from build123d import *

# Parameters (mm, degrees)
BOSS_EXTRUDE1_DEPTH             = 47
SKETCH3_W                       = 84.887301628
SKETCH3_H                       = 42
CUT_EXTRUDE1_DEPTH              = 40
SKETCH4_W                       = 55.556349186
SKETCH4_H                       = 42
CUT_EXTRUDE2_DEPTH              = 10.556349186
SKETCH5_W                       = 55.556349186
SKETCH5_H                       = 42
CUT_EXTRUDE3_DEPTH              = 10.556349186
CUT_EXTRUDE5_REACH              = 130.666
SKETCH7_W                       = 10
SKETCH7_H                       = 18
CUT_EXTRUDE6_REACH              = 135.004
SKETCH8_R                       = 6.5
BOSS_EXTRUDE2_DEPTH             = 5
CUT_EXTRUDE7_REACH              = 105.666
CUT_EXTRUDE7_START              = -5
SKETCH11_W                      = 106
SKETCH11_H                      = 47
BOSS_EXTRUDE3_DEPTH             = 5
CUT_EXTRUDE8_REACH              = 91.961
CUT_EXTRUDE9_REACH              = 91.961
SKETCH14_W                      = 75
SKETCH14_H                      = 27
CUT_EXTRUDE10_REACH             = 136.852
SKETCH16_R                      = 2.1
CUT_EXTRUDE10_DIRECTION_2_DEPTH = 135.851770474
CUT_EXTRUDE11_REACH             = 136.852
SKETCH17_R                      = 2.1


with BuildPart() as part:
    # Sketch1 → Boss-Extrude1 (new body)
    with BuildSketch(Plane(origin=(0, 0, 0), x_dir=(1, 0, 0), z_dir=(0, 1, 0))):
        Polygon((-42.443650814, 0), (42.443650814, 0), (58, 15.556349186), (58, -45), (-58, -45), (-58, 15.556349186), align=None)
    extrude(amount=BOSS_EXTRUDE1_DEPTH)

    # Sketch3 → Cut-Extrude1 (cut)
    with BuildSketch(Plane(origin=(0, 0, 0), x_dir=(-1, 0, 0), z_dir=(0, 0, -1))):
        with Locations((0, 21)):
            Rectangle(SKETCH3_W, SKETCH3_H)
    extrude(amount=-CUT_EXTRUDE1_DEPTH, mode=Mode.SUBTRACT)

    # Sketch4 → Cut-Extrude2 (cut)
    with BuildSketch(Plane.ZY.offset(-42.443650814)):
        with Locations((12.221825407, 21)):
            Rectangle(SKETCH4_W, SKETCH4_H)
    extrude(amount=-CUT_EXTRUDE2_DEPTH, mode=Mode.SUBTRACT)

    # Sketch5 → Cut-Extrude3 (cut)
    with BuildSketch(Plane(origin=(-42.443650814, 0, 0), x_dir=(0, 0, -1), z_dir=(1, 0, 0))):
        with Locations((-12.221825407, 21)):
            Rectangle(SKETCH5_W, SKETCH5_H)
    extrude(amount=-CUT_EXTRUDE3_DEPTH, mode=Mode.SUBTRACT)

    # Sketch7 → Cut-Extrude5 (cut, up to next)
    with BuildSketch(Plane.ZY.offset(-53), mode=Mode.PRIVATE) as cut_extrude5_sk1:
        with Locations((8, 13)):
            Rectangle(SKETCH7_W, SKETCH7_H)
    cut_extrude5_tool1 = extrude(cut_extrude5_sk1.sketch, amount=-CUT_EXTRUDE5_REACH, mode=Mode.PRIVATE) & part.part
    add(cut_extrude5_tool1.solids().sort_by_distance((53, 13, 8))[0], mode=Mode.SUBTRACT)

    # Sketch8 → Cut-Extrude6 (cut, up to next)
    with BuildSketch(Plane.ZY.offset(58), mode=Mode.PRIVATE) as cut_extrude6_sk1:
        with Locations((8.5, 12.301549083)):
            Circle(SKETCH8_R)
    cut_extrude6_tool1 = extrude(cut_extrude6_sk1.sketch, amount=-CUT_EXTRUDE6_REACH, mode=Mode.PRIVATE) & part.part
    add(cut_extrude6_tool1.solids().sort_by_distance((-58, 12.301549, 8.5))[0], mode=Mode.SUBTRACT)

    # Sketch10 → Boss-Extrude2 (add)
    with BuildSketch(Plane(origin=(0, 47, 0), x_dir=(1, 0, 0), z_dir=(0, 1, 0))):
        Polygon((58, -45), (-58, -45), (-58, 15.556349186), (-42.443650814, 0), (42.443650814, 0), (58, 15.556349186), align=None)
    extrude(amount=BOSS_EXTRUDE2_DEPTH)

    # Sketch11 → Cut-Extrude7 (cut, up to next)
    with BuildSketch(Plane.XY.offset(45).offset(CUT_EXTRUDE7_START), mode=Mode.PRIVATE) as cut_extrude7_sk1:
        with Locations((0, 23.5)):
            Rectangle(SKETCH11_W, SKETCH11_H)
    cut_extrude7_tool1 = extrude(cut_extrude7_sk1.sketch, amount=-CUT_EXTRUDE7_REACH, mode=Mode.PRIVATE) & part.part
    add(cut_extrude7_tool1.solids().sort_by_distance((0, 23.5, 40))[0], mode=Mode.SUBTRACT)

    # Sketch12 → Boss-Extrude3 (add)
    with BuildSketch(Plane(origin=(0, 52, 0), x_dir=(1, 0, 0), z_dir=(0, 1, 0))):
        Polygon((58, 15.556349186), (42.443650814, 0), (-42.443650814, 0), (-58, 15.556349186), align=None)
    extrude(amount=-BOSS_EXTRUDE3_DEPTH)

    # Sketch13 → Cut-Extrude8 (cut, up to next)
    with BuildSketch(Plane(origin=(0, 52, 0), x_dir=(1, 0, 0), z_dir=(0, 1, 0)), mode=Mode.PRIVATE) as cut_extrude8_sk1:
        with BuildLine():
            Line((26, 7.556349186), (26, 15.556349186))
            ThreePointArc((26, 15.556349186), (31, 20.556349186), (36, 15.556349186))
            Line((36, 15.556349186), (36, 7.556349186))
            ThreePointArc((36, 7.556349186), (31, 2.556349186), (26, 7.556349186))
        make_face()
    cut_extrude8_tool1 = extrude(cut_extrude8_sk1.sketch, amount=-CUT_EXTRUDE8_REACH, mode=Mode.PRIVATE) & part.part
    # Sketch13 → Cut-Extrude8 (cut, up to next)
    with BuildSketch(Plane(origin=(0, 52, 0), x_dir=(1, 0, 0), z_dir=(0, 1, 0)), mode=Mode.PRIVATE) as cut_extrude8_sk2:
        with BuildLine():
            Line((11.5, 7.556349186), (11.5, 15.556349186))
            ThreePointArc((11.5, 15.556349186), (15, 19.056349186), (18.5, 15.556349186))
            Line((18.5, 15.556349186), (18.5, 7.556349186))
            ThreePointArc((18.5, 7.556349186), (15, 4.056349186), (11.5, 7.556349186))
        make_face()
    cut_extrude8_tool2 = extrude(cut_extrude8_sk2.sketch, amount=-CUT_EXTRUDE8_REACH, mode=Mode.PRIVATE) & part.part
    # Sketch13 → Cut-Extrude8 (cut, up to next)
    with BuildSketch(Plane(origin=(0, 52, 0), x_dir=(1, 0, 0), z_dir=(0, 1, 0)), mode=Mode.PRIVATE) as cut_extrude8_sk3:
        with BuildLine():
            Line((-15.5, 7.556349186), (-15.5, 15.556349186))
            ThreePointArc((-15.5, 15.556349186), (-12, 19.056349186), (-8.5, 15.556349186))
            Line((-8.5, 15.556349186), (-8.5, 7.556349186))
            ThreePointArc((-8.5, 7.556349186), (-12, 4.056349186), (-15.5, 7.556349186))
        make_face()
    cut_extrude8_tool3 = extrude(cut_extrude8_sk3.sketch, amount=-CUT_EXTRUDE8_REACH, mode=Mode.PRIVATE) & part.part
    # Sketch13 → Cut-Extrude8 (cut, up to next)
    with BuildSketch(Plane(origin=(0, 52, 0), x_dir=(1, 0, 0), z_dir=(0, 1, 0)), mode=Mode.PRIVATE) as cut_extrude8_sk4:
        with BuildLine():
            Line((-34.5, 7.556349186), (-34.5, 15.556349186))
            ThreePointArc((-34.5, 15.556349186), (-31, 19.056349186), (-27.5, 15.556349186))
            Line((-27.5, 15.556349186), (-27.5, 7.556349186))
            ThreePointArc((-27.5, 7.556349186), (-31, 4.056349186), (-34.5, 7.556349186))
        make_face()
    cut_extrude8_tool4 = extrude(cut_extrude8_sk4.sketch, amount=-CUT_EXTRUDE8_REACH, mode=Mode.PRIVATE) & part.part
    add(cut_extrude8_tool1.solids().sort_by_distance((31, 52, -11.556349))[0], mode=Mode.SUBTRACT)
    add(cut_extrude8_tool2.solids().sort_by_distance((15, 52, -11.556349))[0], mode=Mode.SUBTRACT)
    add(cut_extrude8_tool3.solids().sort_by_distance((-12, 52, -11.556349))[0], mode=Mode.SUBTRACT)
    add(cut_extrude8_tool4.solids().sort_by_distance((-31, 52, -11.556349))[0], mode=Mode.SUBTRACT)

    # Sketch14 → Cut-Extrude9 (cut, up to next)
    with BuildSketch(Plane(origin=(0, 52, 0), x_dir=(1, 0, 0), z_dir=(0, 1, 0)), mode=Mode.PRIVATE) as cut_extrude9_sk1:
        with Locations((0, -26.5)):
            Rectangle(SKETCH14_W, SKETCH14_H)
    cut_extrude9_tool1 = extrude(cut_extrude9_sk1.sketch, amount=-CUT_EXTRUDE9_REACH, mode=Mode.PRIVATE) & part.part
    add(cut_extrude9_tool1.solids().sort_by_distance((0, 52, 26.5))[0], mode=Mode.SUBTRACT)

    # Sketch16 → Cut-Extrude10 (cut, up to next)
    with BuildSketch(Plane(origin=(58, 0, 0), x_dir=(0, 0, -1), z_dir=(1, 0, 0)), mode=Mode.PRIVATE) as cut_extrude10_sk1:
        with Locations(Location((8.456349186, 10, 0), (0, 0, 180))):
            Circle(SKETCH16_R)
    cut_extrude10_tool1 = extrude(cut_extrude10_sk1.sketch, amount=-CUT_EXTRUDE10_REACH, mode=Mode.PRIVATE) & part.part
    add(cut_extrude10_tool1.solids().sort_by_distance((58, 10, -8.456349))[0], mode=Mode.SUBTRACT)

    # Sketch16 → Cut-Extrude10 direction 2 (cut)
    with BuildSketch(Plane(origin=(58, 0, 0), x_dir=(0, 0, -1), z_dir=(1, 0, 0))):
        with Locations(Location((8.456349186, 10, 0), (0, 0, 180))):
            Circle(SKETCH16_R)
    extrude(amount=CUT_EXTRUDE10_DIRECTION_2_DEPTH, mode=Mode.SUBTRACT)

    # Sketch17 → Cut-Extrude11 (cut, up to next)
    with BuildSketch(Plane.ZY.offset(58), mode=Mode.PRIVATE) as cut_extrude11_sk1:
        with Locations((-8.456349186, 10)):
            Circle(SKETCH17_R)
    cut_extrude11_tool1 = extrude(cut_extrude11_sk1.sketch, amount=-CUT_EXTRUDE11_REACH, mode=Mode.PRIVATE) & part.part
    add(cut_extrude11_tool1.solids().sort_by_distance((-58, 10, -8.456349))[0], mode=Mode.SUBTRACT)


solid = part.part
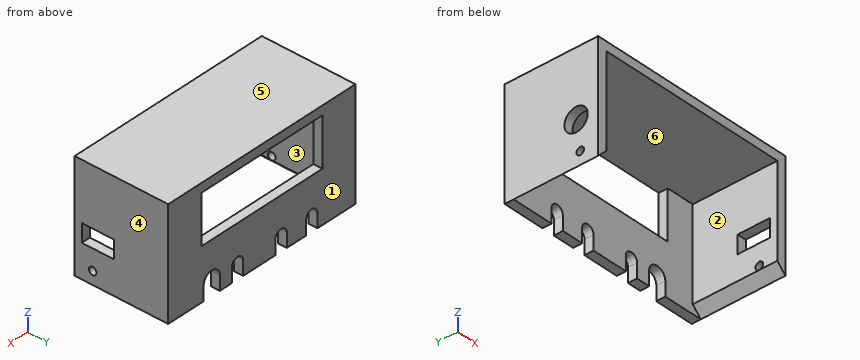
Design review of the part built by this model. Coordinates are the model's own, in mm. Face numbers are marked on the shaded views. A direction names the side the tool comes from. Round coordinates to 2 decimals unless told otherwise and drop trailing zeros. Loops run counter-clockwise (first coordinate to the right, second up) from the corner with the lowest first, then second, coordinate; pieces in that order, holes last. Notation, with made-up numbers: (35, 63) - (68, 63) arc R12 ccw to (68, 73) - close; hole circle Ø5 at (59.25, -9.75). An arc over 180 degrees is marked (long way). One line per item, written item: value. Start each with the question number.
1) Insertion check: pin 1 Ø4 at (x, z) = (44.5, 7.5) entering from -Y; pin 2 Ø6 at (x, y) = (14, 40) entering from -Z; pin 3 Ø2.5 at (x, y) = (54.5, 16) entering from -Z. Each pin has a flat end and moves straight along its axis. Give the tip position at first contact, or say it passes through.
2) Consider section D-D on y = 29. Give the boundary of the cut face in (x, z).
3) For the marked faces 1 and 2, list the 3-axis set-ups (+Z, -Z, +X, -X, +Y, -Y) from which the entire face can be reached by the end or side of a thin tool; tool diameter is ignored.
4) Consider section B-B on x = 15. Give the boundary of the cut face in (y, z), then the cut area to 3 significant figures.
5) Consider section C-C on z = -12. Give the boundary of the cut face in (x, y), then the cut area to 3 significant figures.
6) To check wall thickness, follow L1, parallel to X at y = 30, z = 2.5; L2, parallel to X at y = 50.5, z = 38; L3, parallel to Z at x = 36.5, y = 24. State the ranges of each line that lie inside material, in increasing order. Write a range as from..to.
7) Draft analysis for pull direction X (two halves, no side actions). For the marked faces 3, 4, 5 and 6, state which applies: +X half, -X half, draft (parallel to the pull), parting line (faces both ways), or undercut.
8) Consider section A-A on y = 49. Give the boundary of the cut face in (x, z).
Reported:
1. pin 1: stops at y = 47
1. pin 2: stops at z = 40
1. pin 3: stops at z = -13.31
2. outline: (-58, -15.56) - (-53, -10.56) - (-53, 40) - (53, 40) - (53, -10.56) - (58, -15.56) - (58, 45) - (-58, 45) - close
3. face 1: +Z, -Z, +X, -X, +Y
3. face 2: -Z, -Y
4. outline: (0, 40) - (52, 40) - (52, 45) - (0, 45) - close; (47, -4.06) - (52, -4.06) - (52, 13) - (47, 13) - close
4. area: 345 mm^2
5. outline: (-58, 0) - (-54.44, 0) - (-54.44, 47) - (-34.5, 47) - (-34.5, 52) - (-58, 52) - close; (-27.5, 47) - (-15.5, 47) - (-15.5, 52) - (-27.5, 52) - close; (-8.5, 47) - (11.5, 47) - (11.5, 52) - (-8.5, 52) - close; (18.5, 47) - (26, 47) - (26, 52) - (18.5, 52) - close; (36, 47) - (54.44, 47) - (54.44, 0) - (58, 0) - (58, 52) - (36, 52) - close
5. area: 759 mm^2
6. L1: x = -58..-53, 53..58
6. L2: x = -58..-37.5, 37.5..58
6. L3: z = 40..45
7. face 3: undercut
7. face 4: +X half
7. face 5: draft
7. face 6: undercut
8. outline: (-58, -15.56) - (-34.5, -15.56) - (-34.5, -7.56) arc R3.5 cw to (-27.5, -7.56) - (-27.5, -15.56) - (-15.5, -15.56) - (-15.5, -7.56) arc R3.5 cw to (-8.5, -7.56) - (-8.5, -15.56) - (11.5, -15.56) - (11.5, -7.56) arc R3.5 cw to (18.5, -7.56) - (18.5, -15.56) - (26, -15.56) - (26, -7.56) arc R5 cw to (36, -7.56) - (36, -15.56) - (58, -15.56) - (58, 45) - (-58, 45) - close; hole (-37.5, 13) - (37.5, 13) - (37.5, 40) - (-37.5, 40) - close
